Input: part model. Units: mm. Frame: model coordinates. A direction names the side the tool comes from. Give positions to 0.01 mm unless a question says otherwise; leave off trailing zeros. Write each loop counter-clockwise with the first axis right and the second up, starting at its lowest first coordinate (ties: lowest second). Pieces come first, ordered by that corner, then holes. Notation, with made-up numbers: (75.5, 78) - (84.5, 78) arc R30 cw to (84.5, 107) - close; hole circle Ø2 at (72, 26). An arc over 180 degrees is marked (long way). Use a Markdown table: item, result. Add a question column.
1. Section query D-D, the plane y = 374.5. Return loops of the section in (x, z).
2. Mould query, pull axis X, two halves, no side actions, for faces 3 (the flat face through (637, 352, 0)), 4 (the flat face through (645.694, 351, 1)), 5 (the flat face through (631, 388.42, 1)). Classes: released by +X, released by -X, zero draft, split by the parting line, or undercut.
3. Section query B-B, the plane x = 632.5. Return loops of the section in (y, z), plus the area to 3 significant figures.
4. Material intervals for probe 1 along Y at (x, z) = (628, 2.8); probe 2 along Y at (x, z) = (635.5, 1.8); probe 3 along X at (y, z) = (333, 1.25), sorted ascending.
5. Set-up query: faces 1 (the flat face through (624.694, 316, 1)), 2 (the flat face through (615.694, 351, 1)). Return all of +Z, -Z, +X, -X, +Y, -Y with unobstructed straight access to the full face (end or side cutting, diameter ignored); none if empty.
6. Section query A-A, the plane y = 352.5. Return loops of the section in (x, z).
7. Section query C-C, the plane z = 0.5. Return loops of the section in (x, y), plus the area to 3 significant figures.
```python
from build123d import *

# Parameters (mm, degrees)
SKETCH_1_W      = 30
SKETCH_1_H      = 80
SKETCH_1_R      = 6
SKETCH_1_W_2    = 12
SKETCH_1_H_2    = 3
EXTRUDE_1_DEPTH = 3


with BuildPart() as part:
    # 草图1 → 凸台-拉伸1 (new body)
    with BuildSketch(Plane.XY):
        with Locations((630.693975789, 351.419851644)):
            Rectangle(SKETCH_1_W, SKETCH_1_H)
        with Locations((630.693975789, 351.419851644)):
            Circle(SKETCH_1_R, mode=Mode.SUBTRACT)
        with Locations((630.693975789, 369.419851644)):
            Circle(SKETCH_1_R, mode=Mode.SUBTRACT)
        with Locations((630.693975789, 333.419851644)):
            Circle(SKETCH_1_R, mode=Mode.SUBTRACT)
        with Locations((630.693975789, 315.919851644)):
            Rectangle(SKETCH_1_W_2, SKETCH_1_H_2, mode=Mode.SUBTRACT)
        with Locations((630.693975789, 386.919851644)):
            Rectangle(SKETCH_1_W_2, SKETCH_1_H_2, mode=Mode.SUBTRACT)
    extrude(amount=EXTRUDE_1_DEPTH)


solid = part.part
```
Result sheet:
| question | item | result |
|---|---|---|
| 1 | outline | (615.69, 0) - (627.5, 0) - (627.5, 3) - (615.69, 3) - close; (633.89, 0) - (645.69, 0) - (645.69, 3) - (633.89, 3) - close |
| 2 | face 3 | zero draft |
| 2 | face 4 | released by +X |
| 2 | face 5 | undercut |
| 3 | outline | (311.42, 0) - (314.42, 0) - (314.42, 3) - (311.42, 3) - close; (317.42, 0) - (327.7, 0) - (327.7, 3) - (317.42, 3) - close; (339.14, 0) - (345.7, 0) - (345.7, 3) - (339.14, 3) - close; (357.14, 0) - (363.7, 0) - (363.7, 3) - (357.14, 3) - close; (375.14, 0) - (385.42, 0) - (385.42, 3) - (375.14, 3) - close; (388.42, 0) - (391.42, 0) - (391.42, 3) - (388.42, 3) - close |
| 3 | area | 119 mm² |
| 4 | probe 1 | y = 311.42 to 314.42, 317.42 to 328.06, 338.78 to 346.06, 356.78 to 364.06, 374.78 to 385.42, 388.42 to 391.42 |
| 4 | probe 2 | y = 311.42 to 314.42, 317.42 to 329.83, 337.01 to 347.83, 355.01 to 365.83, 373.01 to 385.42, 388.42 to 391.42 |
| 4 | probe 3 | x = 615.69 to 624.71, 636.68 to 645.69 |
| 5 | face 1 | +Z, -Z |
| 5 | face 2 | +Z, -Z, -X, +Y, -Y |
| 6 | outline | (615.69, 0) - (624.79, 0) - (624.79, 3) - (615.69, 3) - close; (636.6, 0) - (645.69, 0) - (645.69, 3) - (636.6, 3) - close |
| 7 | outline | (615.69, 311.42) - (645.69, 311.42) - (645.69, 391.42) - (615.69, 391.42) - close; hole (624.69, 314.42) - (636.69, 314.42) - (636.69, 317.42) - (624.69, 317.42) - close; hole circle Ø12 at (630.69, 333.42); hole circle Ø12 at (630.69, 351.42); hole circle Ø12 at (630.69, 369.42); hole (624.69, 385.42) - (636.69, 385.42) - (636.69, 388.42) - (624.69, 388.42) - close |
| 7 | area | 1,990 mm² |
